```python
from build123d import *

# Parameters (mm, degrees)
SKETCH_1_W          = 260
SKETCH_1_H          = 55
EXTRUDE_1_DEPTH     = 3
FILLET_1_R          = 3
SKETCH_2_R          = 1.6
CUT_EXTRUDE_1_DEPTH = 48
SKETCH_3_R          = 1.6
SKETCH_3_W          = 80
SKETCH_3_H          = 42
CUT_EXTRUDE_2_DEPTH = 327
FILLET_2_R          = 2


with BuildPart() as part:
    # 草图1 → 凸台-拉伸1 (new body)
    with BuildSketch(Plane.XY):
        Rectangle(SKETCH_1_W, SKETCH_1_H)
    extrude(amount=EXTRUDE_1_DEPTH)

    # 圆角1
    fillet_1_edges = [part.edges().sort_by_distance(p)[0] for p in [
        (-130, 27.5, 1.5),
        (130, 27.5, 1.5),
        (130, -27.5, 1.5),
        (-130, -27.5, 1.5),
    ]]
    fillet(fillet_1_edges, radius=FILLET_1_R)

    # 草图2 → 切除-拉伸1 (cut)
    with BuildSketch(Plane.XY.offset(3)):
        with Locations((-122, 17.5)):
            Circle(SKETCH_2_R)
        with Locations((-122, -2.5)):
            Circle(SKETCH_2_R)
        with Locations((122, -2.5)):
            Circle(SKETCH_2_R)
        with Locations((122, 17.5)):
            Circle(SKETCH_2_R)
    extrude(amount=-CUT_EXTRUDE_1_DEPTH, mode=Mode.SUBTRACT)

    # 草图3 → 切除-拉伸2 (cut)
    with BuildSketch(Plane.XY.offset(3)):
        with Locations((-22, 14.5)):
            Circle(SKETCH_3_R)
        with Locations((-22, -0.5)):
            Circle(SKETCH_3_R)
        with Locations((-22, -15.5)):
            Circle(SKETCH_3_R)
        with Locations((76, 14.5)):
            Circle(SKETCH_3_R)
        with Locations((76, 0)):
            Circle(SKETCH_3_R)
        with Locations((76, -15.5)):
            Circle(SKETCH_3_R)
        with Locations((27, -0.5)):
            Rectangle(SKETCH_3_W, SKETCH_3_H)
    extrude(amount=-CUT_EXTRUDE_2_DEPTH, mode=Mode.SUBTRACT)

    # 圆角2
    fillet_2_edges = [part.edges().sort_by_distance(p)[0] for p in [
        (-13, -21.5, 1.5),
        (-13, 20.5, 1.5),
        (67, 20.5, 1.5),
        (67, -21.5, 1.5),
    ]]
    fillet(fillet_2_edges, radius=FILLET_2_R)


solid = part.part
```
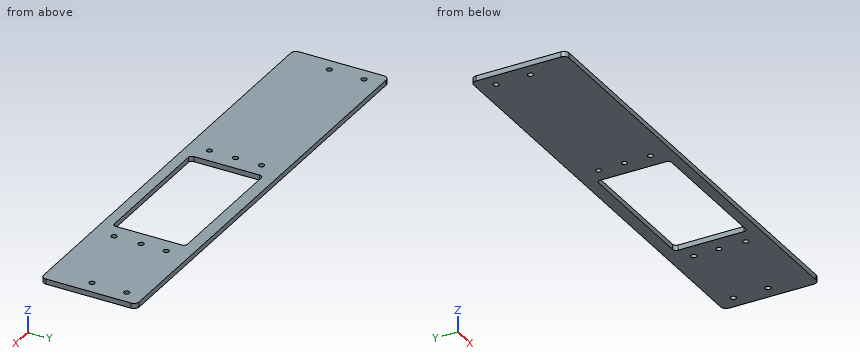
Part model, mm, in its own coordinate system. Round coordinates to 2 decimals unless told otherwise and drop trailing zeros. Loops run counter-clockwise (first coordinate to the right, second up) from the corner with the lowest first, then second, coordinate; pieces in that order, holes last. Notation, with made-up numbers: (88.5, 55.5) -> (132.5, 55.5) arc R18 ccw to (132.5, 61.5) -> close; hole circle Ø11 at (-6, -39.75). An arc over 180 degrees is marked (long way). Use one line per item in the form item = value. Start each with the question number.
Item 1: Band-saw the part on B-B (z = 2.5). Give the number of separate pieces and of enclosed holes in the cut face, plus the area to 3 significant figures.
Item 2: Drop flat-ended pins along their axis: pin 1 Ø3.5 at (x, y) = (76, 14.5) entering from -Z; pin 2 Ø2.5 at (x, y) = (-22, 14.5) entering from +Z. Give the stop position or say it passes through.
Item 3: Band-saw the part on A-A (x = 21). List the corners of the cut face in (y, z), plus the area to 3 significant figures.
Item 4: Drill centre lines: line 1 along Y through (x, z) = (-122, 0.9); line 2 along X through (y, z) = (-9, 0.2); line 3 along Y through (x, z) = (-22, 1.8). Where is each one in solid material? Low to high.
Data:
q1.separate_pieces = 1
q1.enclosed_holes = 11
q1.area = 10,900 mm^2
q2.pin_1 = 0
q2.pin_2 = through
q3.outline = (-27.5, 0) -> (-21.5, 0) -> (-21.5, 3) -> (-27.5, 3) -> close; (20.5, 0) -> (27.5, 0) -> (27.5, 3) -> (20.5, 3) -> close
q3.area = 39.0 mm^2
q4.line_1 = -27.5 to -4.1, -0.9 to 15.9, 19.1 to 27.5
q4.line_2 = -130 to -13, 67 to 130
q4.line_3 = -27.5 to -17.1, -13.9 to -2.1, 1.1 to 12.9, 16.1 to 27.5
